Autodesk Inventor part; units mm, degrees
ref_plane "YZ Plane" through (0, 0, 0) normal (1, 0, 0) x (0, 1, 0)
ref_plane "XZ Plane" through (0, 0, 0) normal (0, 1, 0) x (-1, 0, 0)
ref_plane "XY Plane" through (0, 0, 0) normal (0, 0, 1) x (1, 0, 0)
sketch "Sketch1" plane through (0, 0, 0) normal (0, 0, 1) x (1, 0, 0)
  line L0 (-5.5, 6) -> (5.5, 6)
  line L1 (6, 5.5) -> (6, -5.5)
  line L2 (5.5, -6) -> (-5.5, -6)
  line L3 (-6, -5.5) -> (-6, 5.5)
  line L4 (-6, 6) -> (6, -6) construction
  line L5 (6, 6) -> (-6, -6) construction
  line L6 (-4, 0) -> (4, 0) construction
  line L7 (-4, -0.15) -> (4, -0.15)
  line L8 (4, 0.15) -> (-4, 0.15)
  arc A0 (-4, 0.15) -> (-4, -0.15) centre (-4, 0) ccw
  arc A1 (4, -0.15) -> (4, 0.15) centre (4, 0) ccw
  arc A2 (-5.5, 6) -> (-6, 5.5) centre (-5.5, 5.5) ccw
  arc A3 (-6, -5.5) -> (-5.5, -6) centre (-5.5, -5.5) ccw
  arc A4 (5.5, -6) -> (6, -5.5) centre (5.5, -5.5) ccw
  arc A5 (6, 5.5) -> (5.5, 6) centre (5.5, 5.5) ccw
  point P0 (0, 0)
  dimension "d0" = 12
  dimension "d1" = 12
  dimension "d2" = 4
  dimension "d3" = 0.3
  dimension "d4" = 0.5
extrude "Plate1" add sketch "Sketch1" along normal blind 0.3
equation "\"d5\" = Thickness"
equation "\"BendRadius\" = Thickness"
equation "\"BendReliefWidth\" = Thickness"
equation "\"BendReliefDepth\" = 0.5 * Thickness"
equation "\"CornerReliefSize\" = 4 * Thickness"
equation "\"MinimumRemnant\" = 2 * Thickness"
equation "\"TransitionRadius\" = BendRadius"
equation "\"JacobiRadiusSize\" = BendRadius"
equation "\"GapSize\" = Thickness"
properties part number "Slit" material "Stainless Steel, Austenitic"
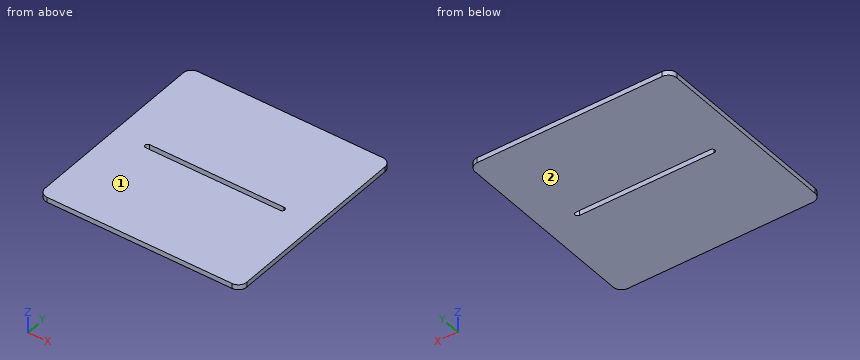
For this review, take the finished solid that the model builds, in its own axes (mm). Face numbers are marked on the shaded views. Coordinates: 2 decimals unless noted, no trailing zeros. Order: outer loops, then holes, each group sorted by start corner. A loop starts at its lowest first (then second) coordinate and runs counter-clockwise, first axis right, second up. Notation, with made-up numbers: (-13.75, 29) - (-2.75, 29) arc R17 ccw to (-2.75, 56) - close; hole circle Ø10 at (-32.5, 72). An arc over 180 degrees is marked (long way). Answer as CSV lines item,"result". Start each with the question number.
1) To check wall thickness, follow line 1 along Y through (x, z) = (3, 0.25). State the ranges of the line that lie inside material, in increasing order. Write a range as [from, to].
2) Add section B-B (z = 0.1). State the section outline as (x, y) points.
3) Add section A-A (y = 0). State the section outline as (x, z) points, then the cut area to 3 significant figures.
4) Add section C-C (x = -0.25). State the section outline as (y, z) points, then the cut area to 3 significant figures.
5) Insertion check: P1, Ø2, axis at x = -4.5, y = -1, coming from the -Z side. The pin has a flat end and moves straight along its axis. Give the tip position at first contact, or say it passes through.
6) Draft analysis for pull direction Z (two halves, no side actions). For the marked faces 1 and 2, state which applies: +Z half, -Z half, draft (parallel to the pull), parting line (faces both ways), or undercut.
Result:
1,line 1,"[-6, -0.15], [0.15, 6]"
2,outline,"(-6, -5.5) arc R0.5 ccw to (-5.5, -6) - (5.5, -6) arc R0.5 ccw to (6, -5.5) - (6, 5.5) arc R0.5 ccw to (5.5, 6) - (-5.5, 6) arc R0.5 ccw to (-6, 5.5) - close; hole (-4, -0.15) - (4, -0.15) arc R0.15 ccw to (4, 0.15) - (-4, 0.15) arc R0.15 ccw to start"
3,outline,"(-6, 0) - (-4.15, 0) - (-4.15, 0.3) - (-6, 0.3) - close; (4.15, 0) - (6, 0) - (6, 0.3) - (4.15, 0.3) - close"
3,area,"1.11 mm^2"
4,outline,"(-6, 0) - (-0.15, 0) - (-0.15, 0.3) - (-6, 0.3) - close; (0.15, 0) - (6, 0) - (6, 0.3) - (0.15, 0.3) - close"
4,area,"3.51 mm^2"
5,P1,"z = 0"
6,face 1,"+Z half"
6,face 2,"-Z half"
